Autodesk Inventor part; units mm, degrees
ref_plane "YZ Plane" through (0, 0, 0) normal (1, 0, 0) x (0, 1, 0)
ref_plane "XZ Plane" through (0, 0, 0) normal (0, 1, 0) x (-1, 0, 0)
ref_plane "XY Plane" through (0, 0, 0) normal (0, 0, 1) x (1, 0, 0)
sketch "Sketch1" plane through (0, 0, 0) normal (1, 0, 0) x (0, 1, 0)
  circle A0 centre (0, -124) radius 1.95
  circle A1 centre (0, 124) radius 1.95
  circle A2 centre (-19, -65) radius 1.5
  circle A3 centre (-19, 65) radius 1.5
  line L0 (0, 124) -> (-19, 65) construction
  line L1 (4.7593, 122.4673) -> (-14.2407, 63.4673)
  line L2 (-23.7593, 66.5327) -> (-4.7593, 125.5327)
  arc A4 (4.7593, 122.4673) -> (-4.7593, 125.5327) centre (0, 124) ccw
  arc A5 (-23.7593, 66.5327) -> (-14.2407, 63.4673) centre (-19, 65) ccw
  line L3 (-19, 65) -> (-19, -65) construction
  line L4 (-24, 65) -> (-24, -65)
  line L5 (-14, -65) -> (-14, 65)
  arc A6 (-14, 65) -> (-24, 65) centre (-19, 65) ccw
  arc A7 (-24, -65) -> (-14, -65) centre (-19, -65) ccw
  line L6 (-19, -65) -> (0, -124) construction
  line L7 (-23.7593, -66.5327) -> (-4.7593, -125.5327)
  line L8 (4.7593, -122.4673) -> (-14.2407, -63.4673)
  arc A8 (-14.2407, -63.4673) -> (-23.7593, -66.5327) centre (-19, -65) ccw
  arc A9 (-4.7593, -125.5327) -> (4.7593, -122.4673) centre (0, -124) ccw
  circle A10 centre (-44, 65) radius 1.5
  circle A11 centre (-44, -65) radius 1.5
  line L9 (-19, 65) -> (-44, 65) construction
  line L10 (-19, 67) -> (-44, 67)
  line L11 (-44, 63) -> (-19, 63)
  arc A12 (-19, 63) -> (-19, 67) centre (-19, 65) ccw
  arc A13 (-44, 67) -> (-44, 63) centre (-44, 65) ccw
  line L12 (-19, -65) -> (-44, -65) construction
  line L13 (-19, -63) -> (-44, -63)
  line L14 (-44, -67) -> (-19, -67)
  arc A14 (-19, -67) -> (-19, -63) centre (-19, -65) ccw
  arc A15 (-44, -63) -> (-44, -67) centre (-44, -65) ccw
  line L15 (0, 124) -> (-44, 65) construction
  line L16 (-4.0081, 126.9891) -> (-48.0081, 67.9891)
  line L17 (-39.9919, 62.0109) -> (4.0081, 121.0109)
  arc A16 (4.0081, 121.0109) -> (-4.0081, 126.9891) centre (0, 124) ccw
  arc A17 (-48.0081, 67.9891) -> (-39.9919, 62.0109) centre (-44, 65) ccw
  line L18 (-44, -65) -> (0, -124) construction
  line L19 (-48.0081, -67.9891) -> (-4.0081, -126.9891)
  line L20 (4.0081, -121.0109) -> (-39.9919, -62.0109)
  arc A18 (-39.9919, -62.0109) -> (-48.0081, -67.9891) centre (-44, -65) ccw
  arc A19 (-4.0081, -126.9891) -> (4.0081, -121.0109) centre (0, -124) ccw
  line L21 (-44, 65) -> (-44, -65) construction
  line L22 (-46.5, 65) -> (-46.5, -65)
  line L23 (-41.5, -65) -> (-41.5, 65)
  arc A20 (-41.5, 65) -> (-46.5, 65) centre (-44, 65) ccw
  arc A21 (-46.5, -65) -> (-41.5, -65) centre (-44, -65) ccw
  line L24 (-44, 65) -> (-19, 0) construction
  line L25 (-45.4, 64.4615) -> (-20.4, -0.5385)
  line L26 (-17.6, 0.5385) -> (-42.6, 65.5385)
  arc A22 (-42.6, 65.5385) -> (-45.4, 64.4615) centre (-44, 65) ccw
  arc A23 (-20.4, -0.5385) -> (-17.6, 0.5385) centre (-19, 0) ccw
  line L27 (-44, -65) -> (-19, 0) construction
  line L28 (-42.6, -65.5385) -> (-17.6, -0.5385)
  line L29 (-20.4, 0.5385) -> (-45.4, -64.4615)
  arc A24 (-45.4, -64.4615) -> (-42.6, -65.5385) centre (-44, -65) ccw
  arc A25 (-17.6, -0.5385) -> (-20.4, 0.5385) centre (-19, 0) ccw
  line L30 (-19, 0) -> (-44, 0) construction
  line L31 (-19, 1.5) -> (-44, 1.5)
  line L32 (-44, -1.5) -> (-19, -1.5)
  arc A26 (-19, -1.5) -> (-19, 1.5) centre (-19, 0) ccw
  arc A27 (-44, 1.5) -> (-44, -1.5) centre (-44, 0) ccw
  circle A28 centre (-19, -10) radius 1.5
  circle A29 centre (-19, -35) radius 1.5
  circle A30 centre (-19, 10) radius 1.5
  circle A31 centre (-19, 35) radius 1.5
  circle A32 centre (0, -124) radius 12.5
  circle A33 centre (0, 124) radius 12.5
  circle A34 centre (-22, 94.5) radius 1
  circle A35 centre (-22, -94.5) radius 1
  circle A36 centre (-11.3392, 88.7888) radius 1
  circle A37 centre (-11.3392, -88.7888) radius 1
  circle A38 centre (-19, 0) radius 1
  point P0 (0, 0)
  point P1 (-9.5, 94.5)
  point P2 (-9.5, -94.5)
  point P3 (-14, -64.2148)
  point P4 (-14, 64.2148)
  point P5 (-24, 65)
  point P6 (-31.5, 65)
  point P7 (-31.5, -65)
  point P8 (-44, 0)
  point P9 (-31.5, 32.5)
  point P10 (-31.5, -32.5)
  point P11 (-41.5, 54.3215)
  point P12 (-24, 8.8215)
  point P13 (-24, 17.1785)
  point P14 (-41.6236, 63)
  point P15 (-24, 63)
  point P16 (-23.6088, 67)
  point P17 (-36.2712, 67)
  point P18 (-13.9854, 96.8832)
  point P19 (-6.8749, 118.9633)
  point P20 (-43.3898, 70)
  point P21 (-46.5, -65)
  point P22 (-43.3898, -70)
  point P23 (-6.8749, -118.9633)
  point P24 (-13.9854, -96.8832)
  point P25 (-36.2712, -67)
  point P26 (-23.6088, -67)
  point P27 (-24, -63)
  point P28 (-41.6236, -63)
  point P29 (-24, -17.1785)
  point P30 (-24, -8.8215)
  point P31 (-41.5, -54.3215)
  point P32 (-31.5, 0)
  point P33 (-41.5, -1.5)
  point P34 (-24, -1.5)
  point P35 (-24, 1.5)
  point P36 (-41.5, 1.5)
  point P37 (-46.5, 60.6699)
  point P38 (-46.5, -60.6699)
  point P39 (-4.0081, -126.9891)
  point P40 (-41.5, 63)
  point P41 (-23.5826, 67)
  point P42 (-41.5, -63)
  point P43 (-41.5, -62.6785)
  point P44 (-41.5, 62.6785)
  point P45 (-10.8571, -117.8053)
  point P46 (1.2475, -111.5624)
  point P47 (-10.8571, 117.8053)
  point P48 (1.2475, 111.5624)
  point P49 (-40.8878, -61.0867)
  point P50 (-41.5, 60.6699)
  dimension "d2" = 3.9
  dimension "d4" = 3.9
  dimension "d25" = 3
  dimension "d28" = 3
  dimension "d43" = 59
  dimension "d44" = 65
  dimension "d45" = 65
  dimension "d47" = 59
  dimension "d48" = 10
  dimension "d49" = 10
  dimension "d50" = 10
  dimension "d52" = 14
  dimension "d53" = 3
  dimension "d54" = 3
  dimension "d55" = 4
  dimension "d56" = 4
  dimension "d57" = 25
  dimension "d58" = 25
  dimension "d59" = 10
  dimension "d60" = 10
  dimension "d61" = 5
  dimension "d62" = 3
  dimension "d63" = 3
  dimension "d64" = 3
  dimension "d65" = 3
  dimension "d66" = 3
  dimension "d67" = 10
  dimension "d68" = 25
  dimension "d69" = 3
  dimension "d70" = 3
  dimension "d71" = 10
  dimension "d72" = 25
  dimension "d73" = 25
  dimension "d74" = 25
  dimension "d76" = 2
  dimension "d78" = 2
  dimension "d79" = 2
  dimension "d80" = 2
  dimension "d81" = 6
  dimension "d82" = 6
  dimension "d83" = 2
extrude "Extrusion1" add sketch "Sketch1" along normal blind 5 contours A4 L16 A33 L1 | A16 L17 A33 L2 A4 | L1 A33 L17 A16 | L1 L5 A6 L10 L2 L17 A33 | A4 L2 A33 L16 | L5 L8 A8 L13 L4 L28 A23 L26 L11 A5 L1 | L1 A5 L11 A12 L10 A6 L5 | L17 L2 A33 | A33 L2 L17 L10 A20 L22 A17 L16 | L8 A32 L20 L7 L14 A7 L5 | L5 A7 L14 A14 L13 A8 L8 | L11 L4 A5 | A5 A6 L10 A12 L11 | A32 L19 A9 L8 | L8 A19 L20 A32 | A6 L2 L10 | L2 A5 L4 L11 L17 L10 | L17 L11 L23 A20 L10 | L22 A20 L10 A13 L25 A17 | A17 L25 L23 L31 A27 L32 L29 A18 L22 | L14 L7 A7 | A7 A8 L13 A14 L14 | A9 L7 A32 L20 A19 | A32 L7 L20 | A8 L4 L13 | A20 L23 L11 L26 A10 L25 A13 L10 | L25 A13 L11 L26 L23 A17 | A17 L23 L25 | L22 A21 L14 L20 L7 A32 L19 A18 | A18 L29 A15 L14 A21 L22 | L26 A25 L31 L25 L4 | L4 L25 L23 A17 L26 | L7 L14 L20 L13 L4 A7 | L19 A32 L7 A9 | L23 L26 L11 | L23 L26 A17 | L25 A10 L26 L11 A13 | L29 L23 A18 | A18 L23 L28 L13 A15 L29 | L25 L31 L4 | A23 L25 L29 A25 | L14 A21 L23 L13 L20 | L28 A18 L23 L29 L4 | L4 L29 L32 A23 L28 | L31 L4 L32 L23 | L23 L32 A27 L31 | A18 L28 L23 | L29 A11 L28 L13 L23 A21 L14 A15 | A15 L13 L28 A11 L29 | L31 L25 L29 L32 L4 | L31 A25 L29 L25 | L4 L32 L29 | L25 A23 L32 L29
sketch "Sketch8" plane through (5, 0, 0) normal (1, 0, 0) x (0, 0, -1)
  line L0 (-54.3215, -41.5) -> (-1.5, -41.5)
  line L1 (-1.5, -41.5) -> (-1.5, -24)
  line L2 (-1.5, -24) -> (-8.8215, -24)
  line L3 (-8.8215, -24) -> (-54.3215, -41.5)
  line L4 (1.5, -24) -> (1.5, -41.5)
  line L5 (1.5, -41.5) -> (54.3215, -41.5)
  line L6 (54.3215, -41.5) -> (8.8215, -24)
  line L7 (8.8215, -24) -> (1.5, -24)
  line L8 (-67, -23.6088) -> (-96.8832, -13.9854)
  line L9 (-96.8832, -13.9854) -> (-67, -36.2712)
  line L10 (-67, -36.2712) -> (-67, -23.6088)
  line L11 (63, -24) -> (17.1785, -24)
  line L12 (17.1785, -24) -> (63, -41.6236)
  line L13 (63, -41.6236) -> (63, -24)
  circle A0 centre (-65, -44) radius 1.5
  circle A1 centre (124, 0) radius 1.95
  circle A2 centre (-124, 0) radius 1.95
  circle A3 centre (-94.5, -22) radius 1
  circle A4 centre (-35, -19) radius 1.5
  circle A5 centre (-10, -19) radius 1.5
  circle A6 centre (35, -19) radius 1.5
  circle A7 centre (10, -19) radius 1.5
  circle A8 centre (65, -19) radius 1.5
  circle A9 centre (88.7888, -11.3392) radius 1
  circle A10 centre (-65, -19) radius 1.5
  circle A11 centre (-88.7888, -11.3392) radius 1
  circle A12 centre (94.5, -22) radius 1
  circle A13 centre (65, -44) radius 1.5
  line L14 (67, -23.6088) -> (67, -36.2712)
  line L15 (67, -36.2712) -> (96.8832, -13.9854)
  line L16 (96.8832, -13.9854) -> (67, -23.6088)
  line L17 (-62.6785, -41.5) -> (-17.1785, -24)
  line L18 (-17.1785, -24) -> (-63, -24)
  line L19 (-63, -24) -> (-63, -41.5)
  line L20 (-63, -41.5) -> (-62.6785, -41.5)
  arc A14 (117.8053, -10.8571) -> (111.5624, 1.2475) centre (124, 0) ccw
  line L21 (117.8053, -10.8571) -> (67.9891, -48.0081)
  arc A15 (60.6699, -46.5) -> (67.9891, -48.0081) centre (65, -44) ccw
  line L22 (60.6699, -46.5) -> (-60.6699, -46.5)
  arc A16 (-67.9891, -48.0081) -> (-60.6699, -46.5) centre (-65, -44) ccw
  line L23 (-67.9891, -48.0081) -> (-117.8053, -10.8571)
  arc A17 (-111.5624, 1.2475) -> (-117.8053, -10.8571) centre (-124, 0) ccw
  line L24 (-111.5624, 1.2475) -> (-64.2148, -14)
  line L25 (-64.2148, -14) -> (64.2148, -14)
  line L26 (64.2148, -14) -> (111.5624, 1.2475)
  circle A18 centre (0, -19) radius 1
  point P0 (0, 0)
sketch "Sketch9" plane through (5, 0, 0) normal (1, 0, 0) x (0, 0, -1)
  circle A0 centre (124, 0) radius 1.95
  circle A1 centre (124, 0) radius 15
  line L0 (111.5624, 1.2475) -> (64.2148, -14)
  circle A2 centre (88.7888, -11.3392) radius 1
  line L1 (67, -23.6088) -> (96.8832, -13.9854)
  line L2 (96.8832, -13.9854) -> (67, -36.2712)
  line L3 (67.9891, -48.0081) -> (117.8053, -10.8571)
  circle A3 centre (94.5, -22) radius 1
  line L4 (71, -11.8149) -> (71, -45.7627)
  circle A4 centre (65, -19) radius 1.5
  point P0 (0, 0)
  point P1 (71, -33.2881)
  point P2 (115.6524, -12.4626)
  point P3 (109.006, 0.4243)
  point P4 (71, -22.3207)
  dimension "d84" = 30
  dimension "d85" = 6
extrude "Extrusion4" add sketch "Sketch9" along normal blind 5 contours A1 L3 L4 L2 L1 L0
sketch "Sketch10" plane through (5, 0, 0) normal (1, 0, 0) x (0, 0, -1)
  line L0 (-181.8877, 79.6872) -> (179.0889, 79.6872)
  line L1 (179.0889, 79.6872) -> (179.0889, -93.8152)
  line L2 (179.0889, -93.8152) -> (-181.8877, -93.8152)
  line L3 (-181.8877, -93.8152) -> (-181.8877, 79.6872)
  point P0 (0, 0)
extrude "Extrusion5" cut sketch "Sketch10" against normal blind 10
properties part number "Horizontal_bar_reinforcement_V2"
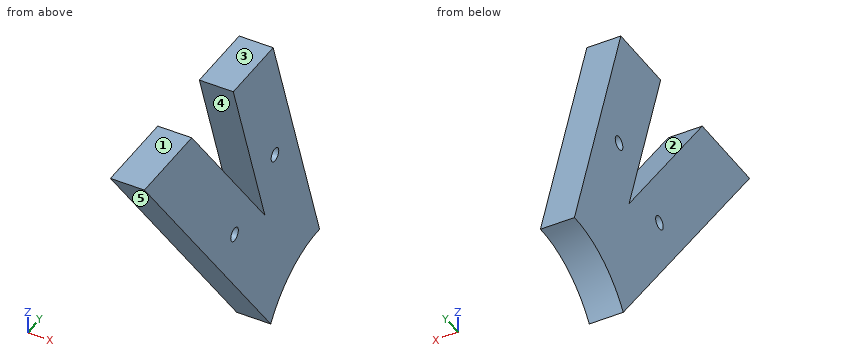
Build history of the part. All positions in model axes, mm. Face numbers are marked on the shaded views. A direction names the side the tool comes from. Round coordinates to 2 decimals unless told otherwise and drop trailing zeros. Loops run counter-clockwise (first coordinate to the right, second up) from the corner with the lowest first, then second, coordinate; pieces in that order, holes last. Notation, with made-up numbers: M 1.25,71 L 21.25,71 A22 ccw 21.25,90 Z; hole C 53.25,-24.5 d4. An arc over 180 degrees is marked long. Answer as CSV lines item,"result".
1. Flat gauge pin, fed straight in: P1, Ø3, axis at x = 8, z = -77, coming from the +Y side. Where does the tip first touch, or does it go through?
Resolved:
P1,"stops at y = -9.4"
2. 3-axis set-ups, long thin cutter, end or side, ignore diameter. For the marked faces 1 and 2: which of +Z, -Z, +X, -X, +Y, -Y reach the whole face in a straight line?
Resolved:
face 1,"+Z, +X, -X, +Y, -Y"
face 2,"+X, -X"
3. Cut at C-C on z = -79. Write the cut outline in (x, y), then the cut area to 3 significant figures.
Resolved:
outline,"M 5,-39.8 L 10,-39.8 L 10,-27.32 L 5,-27.32 Z; M 5,-19.74 L 10,-19.74 L 10,-9.24 L 5,-9.24 Z"
area,"115 mm²"
4. Cut at B-B on x = 8.3. Write the cut outline in (y, z).
Resolved:
outline,"M -45.76,-71 L -12.46,-115.65 A15 cw 0.42,-109.01 L -11.81,-71 L -22.32,-71 L -13.99,-96.88 L -33.29,-71 Z; hole C -22,-94.5 d2; hole C -11.34,-88.79 d2"
5. Two-plate mould, pull along Y, no slides. Class the marked faces 3, 4 and 5: released by +Y, released by -Y, zero draft, split by the parting line, or undercut.
Resolved:
face 3,"zero draft"
face 4,"undercut"
face 5,"released by -Y"
6. Cut at A-A on y = -19. Write the cut outline in (x, z), then the cut area to 3 significant figures.
Resolved:
outline,"M 5,-106.89 L 10,-106.89 L 10,-90.16 L 5,-90.16 Z; M 5,-81.31 L 10,-81.31 L 10,-71 L 5,-71 Z"
area,"135 mm²"
7. Cut at D-D on z = -94.5. Write the cut outline in (x, y), then the cut area to 3 significant figures.
Resolved:
outline,"M 5,-28.24 L 10,-28.24 L 10,-23 L 5,-23 Z; M 5,-21 L 10,-21 L 10,-15.76 L 5,-15.76 Z; M 5,-14.75 L 10,-14.75 L 10,-4.25 L 5,-4.25 Z"
area,"105 mm²"
8. Wall check: probe 1 along Y at (x, z) = (8.2, -94.5); probe 2 along Y at (x, z) = (7.6, -87); probe 3 along Y at (x, z) = (9, -92). Give the ranges that are in metal, low to high. Write a range as [from, to].
Resolved:
probe 1,"y = [-28.24, -23], [-21, -15.76], [-14.75, -4.25]"
probe 2,"y = [-33.83, -21.36], [-17.17, -6.66]"
probe 3,"y = [-30.1, -17.63], [-15.56, -5.05]"
